Input: dimensioned drawing with shaded views. Units: mm. Origin: part minimum x, y, z. Round coordinates to 2 decimals unless told otherwise and drop trailing zeros. Loops run counter-clockwise (first coordinate to the right, second up) from the corner with the lowest first, then second, coordinate; pieces in that order, holes last. Notation, with made-up numbers: (42, -25) - (89, -25) arc R32 ccw to (89, 13) - close; hole circle Ø7 at (51, 27.5). An arc over 180 degrees is marked (long way). One line per question, with ' | ' between items. Start each with the question number.
1. Cut plane A-A (z = 12.5). Return loops of the section in (x, y), then the cut area to 3 significant figures.
2. Pin query (flat end, axial travel): pin 1 (0.8 mm diameter, centred on y = 1.5, z = 11.5, fed in from -X); pin 2 (1.5 mm diameter, centred on x = 4.5, z = 16, fed in from +Y); pin 3 (0.8 mm diameter, centred on x = 11.5, y = 1.5, fed in from -Z). Return the tip coordinate at first contact, or that it passes through.
3. Ray query, line 1 (Z direction, x = 3.25, y = 0.9); line 2 (X direction, y = 1.8, z = 9.75); line 3 (Y direction, x = 17.25, z = 16). Return the intervals inside material, ascending.
4. Cut plane D-D (x = 7.75). Return loops of the section in (y, z), then the cut area to 3 significant figures.
5. Cut plane C-C (z = 5.75). Return loops of the section in (x, y).
6. Cut plane B-B (y = 0.5). Return loops of the section in (x, z).
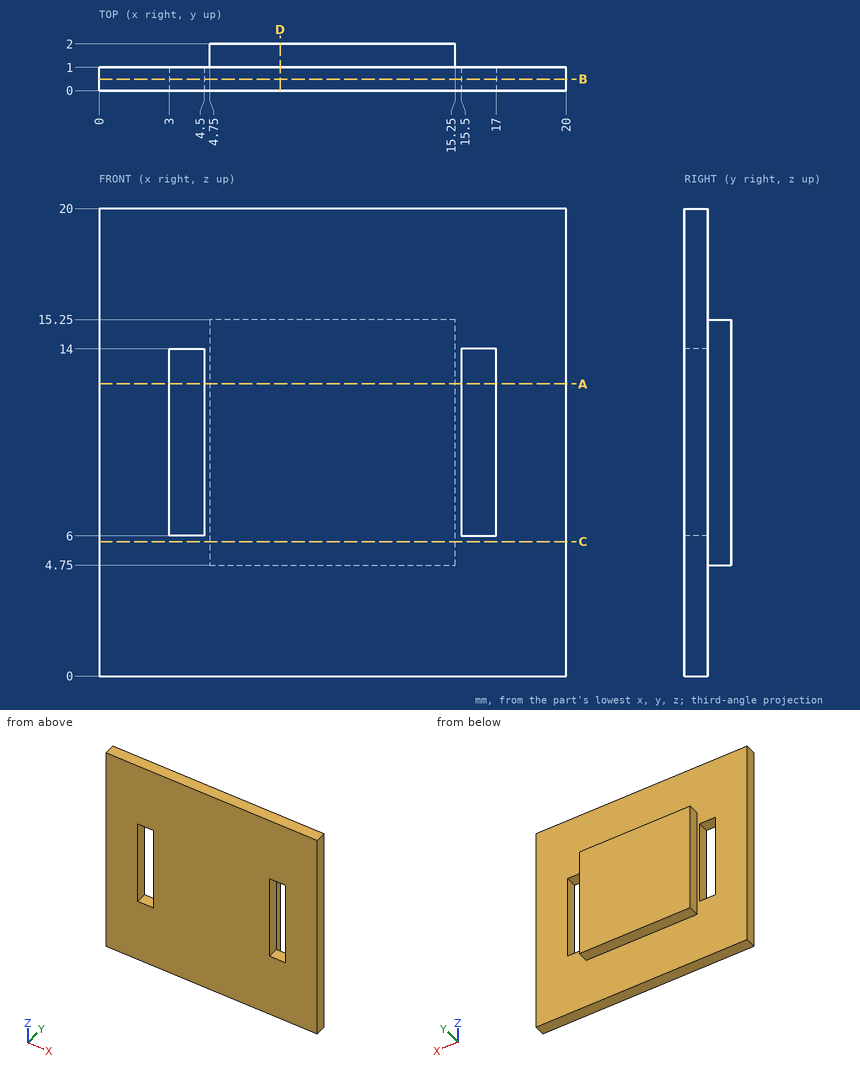
Answers follow:
1) outline: (0, 0) - (3, 0) - (3, 1) - (0, 1) - close; (4.5, 0) - (15.5, 0) - (15.5, 1) - (15.25, 1) - (15.25, 2) - (4.75, 2) - (4.75, 1) - (4.5, 1) - close; (17, 0) - (20, 0) - (20, 1) - (17, 1) - close | area: 27.5 mm2
2) pin 1: stops at x = 4.75 | pin 2: stops at y = 1 | pin 3: stops at z = 4.75
3) line 1: z = 0 to 6, 14 to 20 | line 2: x = 4.75 to 15.25 | line 3: y = 0 to 1
4) outline: (0, 0) - (1, 0) - (1, 4.75) - (2, 4.75) - (2, 15.25) - (1, 15.25) - (1, 20) - (0, 20) - close | area: 30.5 mm2
5) outline: (0, 0) - (20, 0) - (20, 1) - (15.25, 1) - (15.25, 2) - (4.75, 2) - (4.75, 1) - (0, 1) - close
6) outline: (0, 0) - (20, 0) - (20, 20) - (0, 20) - close; hole (3, 6) - (4.5, 6) - (4.5, 14) - (3, 14) - close; hole (15.5, 6) - (17, 6) - (17, 14) - (15.5, 14) - close
